```python
from build123d import *

# Parameters (mm, degrees)
SKETCH1_W                           = 20.5
SKETCH1_H                           = 24.5
BOSS_EXTRUDE1_DEPTH                 = 3.1
SKETCH2_W                           = 5.5
SKETCH2_H                           = 1.1
CUT_EXTRUDE1_DEPTH                  = 29.731142046
SKETCH3_W                           = 16.5
SKETCH3_H                           = 4
BOSS_EXTRUDE2_DEPTH                 = 0.8
TAP_DRILL_FOR_M2_5X0_45_TAP1_REACH  = 22.94
TAP_DRILL_FOR_M2_5X0_45_TAP1_BORE_R = 1.125
TAP_DRILL_FOR_M2X0_4_TAP2_D         = 1.8
FILLET2_R                           = 1


with BuildPart() as part:
    # Sketch1 → Boss-Extrude1 (new body)
    with BuildSketch(Plane(origin=(0, 0, 0), x_dir=(1, 0, 0), z_dir=(0, 1, 0))):
        with Locations((-4.433954619, -2.160858995)):
            Rectangle(SKETCH1_W, SKETCH1_H)
    extrude(amount=BOSS_EXTRUDE1_DEPTH)

    # Sketch2 → Cut-Extrude1 (cut, through all)
    with BuildSketch(Plane.XY.offset(14.410858995)):
        with Locations((3.066045381, 1.55)):
            Rectangle(SKETCH2_W, SKETCH2_H)
    extrude(amount=-CUT_EXTRUDE1_DEPTH, mode=Mode.SUBTRACT)

    # Sketch3 → Boss-Extrude2 (add)
    with BuildSketch(Plane(origin=(0, 3.1, 0), x_dir=(1, 0, 0), z_dir=(0, 1, 0))):
        Polygon((-10.683954619, 10.089141005), (-14.683954619, 10.089141005), (-14.683954619, -14.410858995), (-10.683954619, -14.410858995), (-10.683954619, -10.410858995), (-10.683954619, 6.089141005), align=None)
        with Locations((-2.433954619, 8.089141005)):
            Rectangle(SKETCH3_W, SKETCH3_H)
        with Locations((-2.433954619, -12.410858995)):
            Rectangle(SKETCH3_W, SKETCH3_H)
    extrude(amount=BOSS_EXTRUDE2_DEPTH)

    # Tap Drill for M2.5x0.45 Tap1 bore → Tap Drill for M2.5x0.45 Tap1 (cut, up to next)
    with BuildSketch(Plane(origin=(0, 0, 0), x_dir=(-1, 0, 0), z_dir=(0, -1, 0)), mode=Mode.PRIVATE) as tap_drill_for_m2_5x0_45_tap1_sk1:
        with Locations((-3.066045381, 5.339141005)):
            Circle(TAP_DRILL_FOR_M2_5X0_45_TAP1_BORE_R)
    tap_drill_for_m2_5x0_45_tap1_tool1 = extrude(tap_drill_for_m2_5x0_45_tap1_sk1.sketch, amount=-TAP_DRILL_FOR_M2_5X0_45_TAP1_REACH, mode=Mode.PRIVATE) & part.part
    # Tap Drill for M2.5x0.45 Tap1 bore → Tap Drill for M2.5x0.45 Tap1 (cut, up to next)
    with BuildSketch(Plane(origin=(0, 0, 0), x_dir=(-1, 0, 0), z_dir=(0, -1, 0)), mode=Mode.PRIVATE) as tap_drill_for_m2_5x0_45_tap1_sk2:
        with Locations((-3.066045381, 0.339141005)):
            Circle(TAP_DRILL_FOR_M2_5X0_45_TAP1_BORE_R)
    tap_drill_for_m2_5x0_45_tap1_tool2 = extrude(tap_drill_for_m2_5x0_45_tap1_sk2.sketch, amount=-TAP_DRILL_FOR_M2_5X0_45_TAP1_REACH, mode=Mode.PRIVATE) & part.part
    # Tap Drill for M2.5x0.45 Tap1 bore → Tap Drill for M2.5x0.45 Tap1 (cut, up to next)
    with BuildSketch(Plane(origin=(0, 0, 0), x_dir=(-1, 0, 0), z_dir=(0, -1, 0)), mode=Mode.PRIVATE) as tap_drill_for_m2_5x0_45_tap1_sk3:
        with Locations((-3.066045381, -4.660858995)):
            Circle(TAP_DRILL_FOR_M2_5X0_45_TAP1_BORE_R)
    tap_drill_for_m2_5x0_45_tap1_tool3 = extrude(tap_drill_for_m2_5x0_45_tap1_sk3.sketch, amount=-TAP_DRILL_FOR_M2_5X0_45_TAP1_REACH, mode=Mode.PRIVATE) & part.part
    # Tap Drill for M2.5x0.45 Tap1 bore → Tap Drill for M2.5x0.45 Tap1 (cut, up to next)
    with BuildSketch(Plane(origin=(0, 0, 0), x_dir=(-1, 0, 0), z_dir=(0, -1, 0)), mode=Mode.PRIVATE) as tap_drill_for_m2_5x0_45_tap1_sk4:
        with Locations((-3.046847319, -9.660822138)):
            Circle(TAP_DRILL_FOR_M2_5X0_45_TAP1_BORE_R)
    tap_drill_for_m2_5x0_45_tap1_tool4 = extrude(tap_drill_for_m2_5x0_45_tap1_sk4.sketch, amount=-TAP_DRILL_FOR_M2_5X0_45_TAP1_REACH, mode=Mode.PRIVATE) & part.part
    add(tap_drill_for_m2_5x0_45_tap1_tool1.solids().sort_by_distance((3.066045, 0, -5.339141))[0], mode=Mode.SUBTRACT)
    add(tap_drill_for_m2_5x0_45_tap1_tool2.solids().sort_by_distance((3.066045, 0, -0.339141))[0], mode=Mode.SUBTRACT)
    add(tap_drill_for_m2_5x0_45_tap1_tool3.solids().sort_by_distance((3.066045, 0, 4.660859))[0], mode=Mode.SUBTRACT)
    add(tap_drill_for_m2_5x0_45_tap1_tool4.solids().sort_by_distance((3.046847, 0, 9.660822))[0], mode=Mode.SUBTRACT)

    # Tap Drill for M2x0.4 Tap2 (through all)
    with Locations(Plane(origin=(0, 3.9, 0), x_dir=(1, 0, 0), z_dir=(0, 1, 0))):
        with Locations((-12.683954619, 8.089141005), (-12.674525688, 2.964141005), (-12.764705981, -2.160858995), (-12.764705981, -7.285858995), (-12.764705981, -12.410858995), (-7.558954619, 8.089141005), (-2.433954619, 8.089141005), (-2.514705981, -12.410858995), (-7.639705981, -12.456722912)):
            Hole(TAP_DRILL_FOR_M2X0_4_TAP2_D / 2)

    # Fillet2
    fillet2_edges = [part.edges().sort_by_distance(p)[0] for p in [
        (-14.683954619, 1.95, -10.089141005),
        (-14.683954619, 1.95, 14.410858995),
    ]]
    fillet(fillet2_edges, radius=FILLET2_R)


solid = part.part
```
The listing builds one solid part. Answer for the finished solid, in the listing's coordinates (mm). A direction names the side the tool comes from. Give positions to 0.01 mm unless a question says otherwise; leave off trailing zeros. Order: outer loops, then holes, each group sorted by start corner. A loop starts at its lowest first (then second) coordinate and runs counter-clockwise, first axis right, second up. Notation, with made-up numbers: (48, 64) -> (104, 64) arc R17 ccw to (104, 97) -> close; hole circle Ø4 at (14, 71). An arc over 180 degrees is marked (long way). Answer as CSV lines item,"result". Start each with the question number.
Q1. A cutting plane is placed at D-D (z = -8.5). Determine the outline of the cut face in (x, y).
Q2. A cutting plane is placed at B-B (x = 3.75). Determine the outline of the cut face in (y, z).
Q3. A cutting plane is placed at C-C (x = -7). Determine the outline of the cut face in (y, z).
Q4. Find the intervals of material crossed by L1, parallel to X at y = 2.7, z = -8; L2, parallel to Y at x = 3.5, z = -8.5; L3, parallel to Z at x = -3, y = 0.75, in increasing order.
Q5. Given pin 1 (2 mm diameter, centred on x = 3.07, z = 4.66, fed in from +Y); pin 2 (0.6 mm diameter, centred on y = 3.5, z = 4.5, fed in from +X); pin 3 (2.5 mm diameter, centred on x = -12.76, z = 12.41, fed in from +Y), each flat-ended and moving along its own axis, determine where each tip first touches the part or whether it passes through.
Q6. Determine the mould class of faces 1 (the cylindrical face through (2.461, 0.493, 3.712)), 2 (the flat face through (-4, 2, 14.411)), 3 (the cylindrical face through (-14.4, 1.92, -9.79)) for opening direction X: pulls with the +X half, pulls with the -X half, needs draft (parallel to the pull), parting line crosses it, or undercut.
Q7. A cutting plane is placed at A-A (z = 7.75). Determine the outline of the cut face in (x, y).
Q8. Which of the six approach directions +Z, -Z, +X, -X, +Y, -Y give full straight-line access (tool end or side, diameter ignored) to faces 4 (the cylindrical face through (-13.596, 1.923, 12.756)), 5 (the cylindrical face through (2, 0.5, -0.7)), 6 (the flat face through (3, 1, 2)), 7 (the flat face through (-2.5, 3.5, -6.089)), 8 (the flat face through (-14.684, 2, 2))?
Results found:
1,outline,"(-14.68, 0) -> (-13.48, 0) -> (-13.48, 3.9) -> (-14.68, 3.9) -> close; (-11.88, 0) -> (-8.36, 0) -> (-8.36, 3.9) -> (-11.88, 3.9) -> close; (-6.76, 0) -> (-3.23, 0) -> (-3.23, 3.9) -> (-6.76, 3.9) -> close; (-1.63, 0) -> (5.82, 0) -> (5.82, 1) -> (0.32, 1) -> (0.32, 2.1) -> (5.82, 2.1) -> (5.82, 3.9) -> (-1.63, 3.9) -> close"
2,outline,"(0, -10.09) -> (1, -10.09) -> (1, -6.23) -> (0, -6.23) -> close; (0, -4.45) -> (1, -4.45) -> (1, -1.23) -> (0, -1.23) -> close; (0, 0.55) -> (1, 0.55) -> (1, 3.77) -> (0, 3.77) -> close; (0, 5.55) -> (1, 5.55) -> (1, 8.78) -> (0, 8.78) -> close; (0, 10.54) -> (1, 10.54) -> (1, 14.41) -> (0, 14.41) -> close; (2.1, -10.09) -> (3.9, -10.09) -> (3.9, -6.09) -> (3.1, -6.09) -> (3.1, 10.41) -> (3.9, 10.41) -> (3.9, 14.41) -> (2.1, 14.41) -> close"
3,outline,"(0, -10.09) -> (3.9, -10.09) -> (3.9, -8.79) -> (0, -8.79) -> close; (0, -7.38) -> (3.9, -7.38) -> (3.9, -6.09) -> (3.1, -6.09) -> (3.1, 10.41) -> (3.9, 10.41) -> (3.9, 11.82) -> (0, 11.82) -> close; (0, 13.09) -> (3.9, 13.09) -> (3.9, 14.41) -> (0, 14.41) -> close"
4,L1,"-14.68 to -13.58, -11.79 to -8.45, -6.66 to -3.33, -1.54 to 5.82"
4,L2,"0 to 1, 2.1 to 3.9"
4,L3,"-10.09 to -8.79, -7.39 to 11.65, 13.17 to 14.41"
5,pin 1,"y = 3.1"
5,pin 2,"x = -10.68"
5,pin 3,"y = 3.9"
6,face 1,"undercut"
6,face 2,"needs draft"
6,face 3,"pulls with the -X half"
7,outline,"(-14.68, 0) -> (-13.54, 0) -> (-13.54, 3.9) -> (-14.68, 3.9) -> close; (-11.99, 0) -> (5.82, 0) -> (5.82, 1) -> (0.32, 1) -> (0.32, 2.1) -> (5.82, 2.1) -> (5.82, 3.1) -> (-10.68, 3.1) -> (-10.68, 3.9) -> (-11.99, 3.9) -> close"
8,face 4,"+Y, -Y"
8,face 5,"-Y"
8,face 6,"+Z, -Z, +X"
8,face 7,"+X, +Y"
8,face 8,"+Z, -Z, -X, +Y, -Y"
